The model under review builds one solid part; all positions refer to its coordinate system, in mm. Face numbers are marked on the shaded views. A direction names the side the tool comes from. Coordinates: 2 decimals unless noted, no trailing zeros. Order: outer loops, then holes, each group sorted by start corner. A loop starts at its lowest first (then second) coordinate and runs counter-clockwise, first axis right, second up.
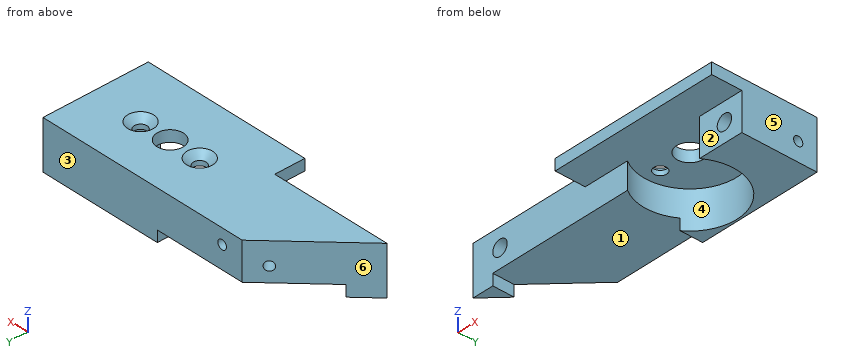
Autodesk Inventor part; units mm, degrees
ref_plane "YZ Plane" through (0, 0, 0) normal (1, 0, 0) x (0, 1, 0)
ref_plane "XZ Plane" through (0, 0, 0) normal (0, 1, 0) x (-1, 0, 0)
ref_plane "XY Plane" through (0, 0, 0) normal (0, 0, 1) x (1, 0, 0)
sketch "Sketch1" plane through (0, 0, 0) normal (0, 1, 0) x (-1, 0, 0)
  line L0 (0, 0) -> (81.5, 0)
  line L1 (81.5, 0) -> (81.5, -13)
  line L2 (81.5, -13) -> (0, -13)
  line L3 (0, -13) -> (0, 0)
  dimension "d0" = 81.5
  dimension "d1" = 13
extrude "Extrusion1" add sketch "Sketch1" along normal blind 30
sketch "Sketch2" plane through (0, 0, -13) normal (0, 0, -1) x (-1, 0, 0)
  line L0 (0, 0) -> (0, 30)
  line L1 (0, 0) -> (81.5086, 0)
  line L2 (81.5086, 0) -> (81.5086, 8)
  line L3 (81.5086, 8) -> (0, 8)
  line L4 (0, 8) -> (0, 0)
  line L5 (81.5, 0) -> (81.5, 30)
  line L6 (81.5, 0) -> (22.5, 0)
  line L7 (0, 0) -> (81.5, 0)
  line L8 (22.5, 0) -> (22.5, 15)
  circle A0 centre (22.5, 15) radius 12.5
  dimension "d4" = 81.5086
  dimension "d5" = 8
  dimension "d6" = 59
  dimension "d7" = 15
  dimension "d8" = 25
extrude "Extrusion2" cut sketch "Sketch2" against normal blind 10
sketch "Sketch3" plane through (-81.5, 0, 0) normal (0, 0, 1) x (1, 0, 0)
  line L0 (0, 8) -> (0, 30)
  line L1 (0, 30) -> (0, 8)
  line L2 (0, 30) -> (22, 30)
  line L3 (0, 30) -> (81.5, 30)
  line L4 (22, 30) -> (0, 8)
  line L5 (81.5, 0) -> (81.5, 8)
  line L6 (81.5, 0) -> (36.5, 0)
  line L7 (0, 0) -> (81.5, 0)
  line L8 (48.6438, 8) -> (0, 8)
  line L9 (36.5, 0) -> (0, 0)
  line L10 (0, 0) -> (0, 8)
  line L11 (0, 8) -> (36.5, 8)
  line L12 (36.5, 8) -> (36.5, 0)
  dimension "d11" = 22
  dimension "d12" = 45
extrude "Extrusion3" cut sketch "Sketch3" against normal blind 13
sketch "Sketch4" plane through (0, 30, 0) normal (0, 1, 0) x (1, 0, 0)
  line L0 (0, 0) -> (0, 13)
  line L1 (-59.5, 0) -> (-81.5, 0)
  line L2 (0, 13) -> (-81.5, 13)
  line L3 (-81.5, 13) -> (-81.5, 0)
  line L4 (-81.5, 0) -> (0, 0)
  line L5 (0, 0) -> (0, 13)
extrude "Extrusion4" cut sketch "Sketch4" against normal blind 2
sketch "Sketch6" plane through (0, 0, -3) normal (0, 0, -1) x (-1, 0, 0)
  arc A0 (32.8562, 8) -> (12.1438, 8) centre (22.5, 15) ccw
  circle A1 centre (22.5, 15) radius 3.5
  point P0 (0, 0)
  dimension "d17" = 7
extrude "Extrusion5" cut sketch "Sketch6" against normal blind 3
sketch "Sketch7" plane through (-45, 0, 0) normal (0, 0, 1) x (1, 0, 0)
  circle A0 centre (22.5, 15) radius 3.5
  line L0 (22.5, 15) -> (31, 15)
  line L1 (22.5, 15) -> (14, 15)
  point P0 (45, 0)
  dimension "d20" = 8.5
  dimension "d21" = 8.5
hole "Hole1" at (-14, 15, 0) at (-31, 15, 0) direction (0, 0, -1) diameter 3.4 end through all countersink diameter 6.9 countersink angle 89.954
sketch "Sketch8" plane through (-32.8562, 8, -13) normal (0, -1, 0) x (1, 0, 0)
  line L0 (0, 0) -> (-48.6438, 0)
  line L1 (-48.6438, 0) -> (-36.6438, 0)
  line L2 (-36.6438, 0) -> (-36.6438, 8)
  line L3 (32.8562, 10) -> (32.8562, 0)
  line L4 (32.8562, 0) -> (32.8562, 5)
  line L5 (32.8562, 5) -> (27.8562, 5)
  point P0 (32.8562, 13)
  dimension "d82" = 8
  dimension "d83" = 5
  dimension "d84" = 5
hole "Hole2" at (-5, 8, -8) at (-69.5, 8, -5) direction (0, 1, 0) diameter 4.134 depth 5.6 tip angle 118
sketch "Sketch9" plane through (0, 0, 0) normal (1, 0, 0) x (0, 0, -1)
  line L0 (8, 28) -> (8, 23)
  line L1 (0, 28) -> (13, 28)
  line L2 (8, 28) -> (13, 28)
  point P0 (0, 0)
  point P1 (13, 8)
  dimension "d40" = 5
hole "Hole3" at (0, 23, -8) direction (-1, 0, 0) diameter 2.459 depth 9 tip angle 118
sketch "Sketch10" plane through (0, 28, 0) normal (0, 1, 0) x (1, 0, 0)
  line L0 (-61.5, 0) -> (-61.5, 13)
  line L1 (-61.5, 0) -> (-61.5, 4)
  line L2 (-61.5, 4) -> (-51.5, 4)
  point P0 (0, 0)
  dimension "d76" = 4
  dimension "d77" = 10
hole "Hole4" at (-51.5, 28, -4) direction (0, -1, 0) diameter 2.459 depth 9 tip angle 118
sketch "Sketch12" plane through (-45, 0, 0) normal (0, 0, 1) x (1, 0, 0)
  line L0 (12.1438, 8) -> (-36.5, 8)
  line L1 (-36.5, 8) -> (-33.5, 8)
  line L2 (-16.5, 28) -> (45, 28)
  line L3 (-16.5, 28) -> (-13.5, 28)
  line L4 (-13.5, 28) -> (-33.5, 8)
  line L5 (-36.5, 8) -> (-16.5, 28)
  line L6 (-13.5, 28) -> (-12.257, 28)
  line L7 (45, 28) -> (-16.5, 28)
  line L8 (-12.257, 28) -> (-32.257, 8)
  line L9 (-33.5, 8) -> (-32.257, 8)
  point P0 (45, 0)
  dimension "d71" = 3
  dimension "d72" = 3
  dimension "d75" = 1.243
extrude "Extrusion6" cut sketch "Sketch12" against normal blind 25.4
sketch "Sketch13" plane through (-22.5, 15, -13) normal (0, 0, -1) x (-1, 0, 0)
  line L0 (10.3562, -7) -> (54.757, -7)
  line L1 (10.3562, -7) -> (47.3562, -7)
  line L2 (47.3562, -7) -> (47.3562, 0.4008)
  line L3 (34.757, 13) -> (54.757, -7)
  line L4 (34.757, 13) -> (-22.5, 13)
  line L5 (47.3562, 0.4008) -> (34.757, 13)
  line L6 (34.757, 13) -> (10.3562, 13)
  arc A0 (10.3562, -7) -> (-10.3562, -7) centre (0, 0) ccw
  line L7 (10.3562, -7) -> (10.3562, 13)
  line L8 (49.067, -7) -> (44.933, -7)
  line L9 (47.3562, -7) -> (49.067, -7)
  line L10 (49.067, -7) -> (49.067, -1.31)
  line L11 (47.3562, 0.4008) -> (49.067, -1.31)
  line L12 (54.757, -7) -> (34.757, 13)
  point P0 (-22.5, -15)
  dimension "d79" = 37
extrude "Extrusion7" cut sketch "Sketch13" against normal blind 3 contours A0 L7 L4 L3 L2 L0 | L7 A0 | L2 L3 L10 L0
sketch "Sketch11" plane through (-79.3785, 5.8785, -13) normal (-0.7071068, 0.7071068, 0) x (-0.7071068, -0.7071068, 0)
  line L0 (-31.2845, 3) -> (-31.2845, 13)
  line L1 (-3.0003, 0) -> (-11.0471, 0)
  point P0 (-51.9723, 13)
  point P1 (-25.9845, 7)
  dimension "d111" = 5.3
  dimension "d112" = 7
hole "Hole5" at (-61.0047, 24.2523, -6) direction (0.7071068, -0.7071068, 0) diameter 2.459 depth 10 tip angle 118
properties part number "mocowanie_silnika_wariant1"
(1) We need section B-B, the plane x = -31. Write out the cut boundary in (y, z), and give its area (3 significant figures).
A:
outline: (0, -3) - (13.3, -3) - (13.3, -1.75) - (11.55, 0) - (0, 0) - close; (16.7, -3) - (24.17, -3) - (24.17, -13) - (28, -13) - (28, 0) - (18.45, 0) - (16.7, -1.75) - close
area: 109 mm2
(2) Wall thickness on probe 1 along Z at (x, y) = (-69.5, 10.4); probe 2 along X at (y, z) = (14, -8.25): over which ranges is each line inside the solid? List them lowest first.
A:
probe 1: z = -10 to -7.07, -2.93 to 0
probe 2: x = -71.26 to -34.96, -10.04 to -6.38, -3.62 to 0
(3) Draft analysis for pull direction Y (two halves, no side actions). For the marked faces 4, 5 and 6, state which applies: released by +Y, released by -Y, zero draft, split by the parting line, or undercut.
A:
face 4: undercut
face 5: zero draft
face 6: released by +Y
(4) We need section C-C, the plane y = 6. Write out the cut boundary in (x, z).
A:
outline: (-45, -3) - (0, -3) - (0, 0) - (-45, 0) - close
(5) We need section A-A, the plane z = -10.75. Write out the cut boundary in (x, y).
A:
outline: (-77.26, 8) - (-71.57, 8) - (-71.57, 13.69) - close; (-32.86, 22) arc R12.5 cw to (-12.14, 8) - (0, 8) - (0, 28) - (-32.86, 28) - close
(6) Machinability: for the marked faces 1, 2 and 3, which of the approach directions +Z, -Z, +X, -X, +Y, -Y give a long, thin tool a straight path to every point of the face, cutting with its end or side? Answer none if there is none.
A:
face 1: -Z, +Y, -Y
face 2: -Z, +X, -X, -Y
face 3: +Z, -Z, +X, -X, +Y
(7) For pin 1 Ø6.5 at (x, z) = (-69.5, -5) entering from +Y; pin 2 Ø3.5 at (y, z) = (25, -12) entering from -X; pin 3 Ø0.9 at (y, z) = (3.5, -2) entering from -X, all flat-tipped, find the tip position at first contact; note any pin that passes through.
A:
pin 1: stops at y = 19.01
pin 2: stops at x = -32.86
pin 3: stops at x = -45
